Autodesk Inventor part; units mm, degrees
ref_plane "YZ Plane" through (0, 0, 0) normal (1, 0, 0) x (0, 1, 0)
ref_plane "XZ Plane" through (0, 0, 0) normal (0, 1, 0) x (-1, 0, 0)
ref_plane "XY Plane" through (0, 0, 0) normal (0, 0, 1) x (1, 0, 0)
sketch "草图1" plane through (0, 0, 0) normal (0, 1, 0) x (-1, 0, 0)
  line L0 (68.3073, 0) -> (21.1081, -64.9641)
  line L1 (21.1081, -64.9641) -> (-55.2617, -40.15)
  line L2 (-55.2617, -40.15) -> (-55.2617, 40.15)
  line L3 (-55.2617, 40.15) -> (21.1081, 64.9641)
  line L4 (21.1081, 64.9641) -> (68.3073, 0)
  line L5 (105.0554, 0) -> (32.4639, -99.9136)
  line L6 (32.4639, -99.9136) -> (-84.9916, -61.75)
  line L7 (-84.9916, -61.75) -> (-84.9916, 61.75)
  line L8 (-84.9916, 61.75) -> (32.4639, 99.9136)
  line L9 (32.4639, 99.9136) -> (105.0554, 0)
  point P0 (0, 0)
  point P1 (0, 0)
  point P2 (0, 0)
  dimension "d0" = 80.3
  dimension "d1" = 123.5
extrude "拉伸1" add sketch "草图1" along normal blind 2
sketch "草图2" plane through (0, 2, 0) normal (0, 1, 0) x (1, 0, 0)
  line L0 (-21.1081, 64.9641) -> (55.2617, 40.15)
  line L1 (55.2617, 40.15) -> (55.2617, -40.15)
  line L2 (55.2617, -40.15) -> (-21.1081, -64.9641)
  line L3 (-21.1081, -64.9641) -> (-68.3073, 0)
  line L4 (-68.3073, 0) -> (-21.1081, 64.9641)
  line L5 (-32.4639, 99.9136) -> (-105.0554, 0)
  line L6 (-105.0554, 0) -> (-32.4639, -99.9136)
  line L7 (-32.4639, -99.9136) -> (84.9916, -61.75)
  line L8 (84.9916, -61.75) -> (84.9916, 61.75)
  line L9 (84.9916, 61.75) -> (-32.4639, 99.9136)
  line L10 (58.7617, 42.6929) -> (-22.445, 69.0786)
  line L11 (-22.445, 69.0786) -> (-72.6335, 0)
  line L12 (-72.6335, 0) -> (-22.445, -69.0786)
  line L13 (-22.445, -69.0786) -> (58.7617, -42.6929)
  line L14 (58.7617, -42.6929) -> (58.7617, 42.6929)
  line L15 (-23.2089, 71.4297) -> (60.7617, 44.146)
  line L16 (60.7617, 44.146) -> (60.7617, -44.146)
  line L17 (60.7617, -44.146) -> (-23.2089, -71.4297)
  line L18 (-23.2089, -71.4297) -> (-75.1056, 0)
  line L19 (-75.1056, 0) -> (-23.2089, 71.4297)
  point P0 (0, 0)
  dimension "d4" = 3.5
  dimension "d5" = 2
extrude "拉伸2" add sketch "草图2" along normal blind 10 contours L15 L16 L17 L18 L19
sketch "草图3" plane through (0, 0, 0) normal (0, -1, 0) x (1, 0, 0)
  line L0 (-9.4145, -72.1274) -> (53.3776, -50.8644)
  line L1 (53.3776, -50.8644) -> (57.7542, -63.7889)
  line L2 (57.7542, -63.7889) -> (-5.038, -85.0518)
  line L3 (-5.038, -85.0518) -> (-9.4145, -72.1274)
  point P0 (0, 0)
extrude "拉伸3" cut sketch "草图3" against normal blind 10
sketch "草图4" plane through (0, 0, 0) normal (0, -1, 0) x (1, 0, 0)
  line L0 (-105.0554, 0) -> (-32.4639, -99.9136)
  line L1 (-105.0554, 0) -> (0, 0)
  line L2 (0, 0) -> (99.3977, 72.2167)
  line L3 (99.3977, 72.2167) -> (-62.0091, 125.592)
  line L4 (-62.0091, 125.592) -> (-127.7953, 9.1282)
  line L5 (-127.7953, 9.1282) -> (-105.0554, 0)
extrude "拉伸4" cut sketch "草图4" against normal blind 16.75 keep common part
properties part number "上部端盖" material "橡胶"
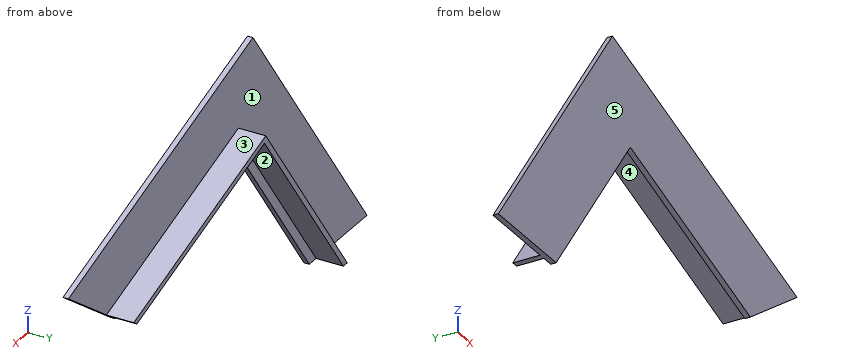
Geometry: final body of the model. Coordinates: model frame, mm. Face numbers are marked on the shaded views. A direction names the side the tool comes from. Give positions to 0.01 mm unless a question says otherwise; leave off trailing zeros. Write each loop counter-clockwise with the first axis right and the second up, starting at its lowest first coordinate (ties: lowest second). Pieces come first, ordered by that corner, then holes. Notation, with made-up numbers: M 50.5,61.25 L 86.5,61.25 A30 cw 86.5,95.25 Z; hole C 33.5,-2 d8. An arc over 180 degrees is marked long. Answer in a Markdown table with one row per item. Add a question column.
(1) Reachability of the marked faces 1 and 2 from +Z, -Z, +X, -X, +Y, -Y: full face, straight path, thin tool, end or side. Return the list, or none.
(2) Section C-C on z = 81.5. Return loops of the section in (x, y).
(3) Section D-D on x = 24. Return loops of the section in (y, z).
(4) Ray query, line 1 (Y direction, x = -4.5, z = 60); line 2 (Z direction, x = 35, y = 3.75); line 3 (X direction, y = 3.5, z = 41). Return the intervals inside material, ascending.
(5) Section B-B on x = -45.5. Return loops of the section in (y, z), and give its area (3 significant figures).
(6) First-contact query: pin 1 (1.5 mm diameter, centred on y = 10, z = 30.5, fed in from +X); pin 2 (1.5 mm diameter, centred on y = 7.5, z = 60.5, fed in from -X); pin 3 (6 mm diameter, centred on x = -28.5, y = 6, fed in from +Z). Flat tips, straight axial feed; report the tip coordinate or a pass-through.
(7) Mould query, pull axis X, two halves, no side actions, for the marked faces 3, 4 and 5. Classes: +X half, -X half, draft (parallel to the pull), parting line (faces both ways), or undercut.
Result set:
| question | item | result |
|---|---|---|
| 1 | face 1 | +Z, +Y |
| 1 | face 2 | -Z, +Y |
| 2 | outline | M -45.84,0 L 24.21,0 L 24.21,2 L -45.84,2 Z |
| 3 | outline | M 0,50.31 L 2,50.31 L 2,53.99 L 12,53.99 L 12,56.09 L 2,56.09 L 2,81.57 L 0,81.57 Z |
| 4 | line 1 | y = 0 to 2 |
| 4 | line 2 | z = 50.41 to 52.52 |
| 4 | line 3 | x = -45.32 to -42.85 |
| 5 | outline | M 0,31.39 L 2,31.39 L 2,37.35 L 12,37.35 L 12,40.75 L 2,40.75 L 2,81.97 L 0,81.97 Z |
| 5 | area | 135 mm^2 |
| 6 | pin 1 | stops at x = -49.93 |
| 6 | pin 2 | stops at x = -31.69 |
| 6 | pin 3 | stops at z = 68.28 |
| 7 | face 3 | +X half |
| 7 | face 4 | undercut |
| 7 | face 5 | draft |
